```python
from build123d import *

# Parameters (mm, degrees)
BOSS_EXTRUDE2_DEPTH      = 1.5875
BOSS_EXTRUDE2_DEPTH_BACK = 1.5875
SKETCH4_R                = 1.1
FILLET2_R                = 2.54


with BuildPart() as part:
    # Sketch4 → Boss-Extrude2 (new, two sides: drawn at the far end of the back side and taken through both)
    with BuildSketch(Plane(origin=(0, 0, 41.275), x_dir=(-1, 0, 0), z_dir=(0, 0, -1)).offset(-BOSS_EXTRUDE2_DEPTH_BACK)):
        Polygon((205.973378569, 28.316894771), (215.496993412, 28.479330378), (215.442840335, 31.654330378), (259.682693032, 44.354330378), (259.886376268, 32.412363209), (259.940529345, 29.237363209), (269.464144188, 29.399798816), (269.51828939, 26.225260535), (206.027523772, 25.14235649), align=None)
        with Locations((254.716415099, 37.643475636)):
            Circle(SKETCH4_R, mode=Mode.SUBTRACT)
    extrude(amount=BOSS_EXTRUDE2_DEPTH + BOSS_EXTRUDE2_DEPTH_BACK)

    # Fillet2
    fillet2_edges = [part.edges().sort_by_distance(p)[0] for p in [
        (-259.682693032, 44.354330378, 41.275),
    ]]
    fillet(fillet2_edges, radius=FILLET2_R)


solid = part.part
```
Geometry check sheet. Reference: the model listing, model coordinates, mm. Give positions to 0.01 mm unless a question says otherwise; leave off trailing zeros. Order: outer loops, then holes, each group sorted by start corner. A loop starts at its lowest first (then second) coordinate and runs counter-clockwise, first axis right, second up. Notation, with made-up numbers: (-4.75, -12.5) - (33.25, -12.5) arc R12 cw to (33.25, 1.5) - close; hole circle Ø7 at (-10, -3). An arc over 180 degrees is marked (long way). Answer in a Markdown table with one row per item. Add a question column.
Q1. Cross-section at B-B, the plane y = 33.5. Enter the section's corners in (x, z), then the cut area to 3 significant figures.
Q2. Material ranges on probe 1 along Y at (x, z) = (-254, 42.05); probe 2 along Y at (x, z) = (-222, 40.05); probe 3 along X at (y, z) = (26.5, 40.85), recorded low to high. Write a range as from..to.
Q3. Cross-section at A-A, the plane z = 42.2. Enter the section's corners in (x, y).
Q4. Cross-section at C-C, the plane x = -242. Enter the section's corners in (y, z).
Q5. Mould release check, pull along X, two halves, no side actions. Record for faces 1 (the cylindrical face through (-258.684, 43.06, 41.253)), 2 (the cylindrical face through (-253.617, 37.692, 41.297)), 3 (the flat face through (-235.683, 37.465, 41.297)), 4 (the flat face through (-245, 32, 42.862)): pulls with the +X half, pulls with the -X half, needs draft (parallel to the pull), parting line crosses it, or undercut.
Q6. Gauge pin test, flat ends, axial feed: pin 1 (1.8 mm diameter, centred on x = -254.72, y = 37.64, fed in from +Z); pin 2 (10 mm diameter, centred on x = -230, y = 41, fed in from +Z). Record the tip position at first contact, or that the pin passes through.
Check values:
| question | item | result |
|---|---|---|
| 1 | outline | (-259.87, 39.69) - (-221.87, 39.69) - (-221.87, 42.86) - (-259.87, 42.86) - close |
| 1 | area | 121 mm^2 |
| 2 | probe 1 | y = 25.96..36.81, 38.48..42.72 |
| 2 | probe 2 | y = 25.41..33.54 |
| 2 | probe 3 | x = -269.51..-206 |
| 3 | outline | (-269.52, 26.23) - (-206.03, 25.14) - (-205.97, 28.32) - (-215.5, 28.48) - (-215.44, 31.65) - (-256.5, 43.44) arc R2.54 ccw to (-259.74, 41.04) - (-259.94, 29.24) - (-269.46, 29.4) - close; hole circle Ø2.2 at (-254.72, 37.64) |
| 4 | outline | (25.76, 39.69) - (39.28, 39.69) - (39.28, 42.86) - (25.76, 42.86) - close |
| 5 | face 1 | parting line crosses it |
| 5 | face 2 | undercut |
| 5 | face 3 | pulls with the +X half |
| 5 | face 4 | needs draft |
| 6 | pin 1 | passes through |
| 6 | pin 2 | stops at z = 42.86 |
